```python
from build123d import *

# Parameters (mm, degrees)
SKETCH1_W           = 25
SKETCH1_H           = 35
SKETCH1_R           = 4
BOSS_EXTRUDE1_DEPTH = 6
FILLET1_R           = 12.5
SKETCH2_R           = 20
CUT_EXTRUDE1_DEPTH  = 6


with BuildPart() as part:
    # Sketch1 → Boss-Extrude1 (new body)
    with BuildSketch(Plane(origin=(0, 0, 0), x_dir=(1, 0, 0), z_dir=(0, 1, 0))):
        with Locations((12.5, 17.5)):
            Rectangle(SKETCH1_W, SKETCH1_H)
        with Locations(Location((12.5, 25, 0), (0, 0, 270))):
            Circle(SKETCH1_R, mode=Mode.SUBTRACT)
    extrude(amount=BOSS_EXTRUDE1_DEPTH)

    # Fillet1
    fillet1_edges = [part.edges().sort_by_distance(p)[0] for p in [
        (25, 3, -35),
        (0, 3, -35),
    ]]
    fillet(fillet1_edges, radius=FILLET1_R - 0.0001)  # a hair under: the kernel refuses the full size

    # Sketch2 → Cut-Extrude1 (cut)
    with BuildSketch(Plane(origin=(0, 6, 0), x_dir=(1, 0, 0), z_dir=(0, 1, 0))):
        with Locations((12.5, -12)):
            Circle(SKETCH2_R)
    extrude(amount=-CUT_EXTRUDE1_DEPTH, mode=Mode.SUBTRACT)


solid = part.part
```
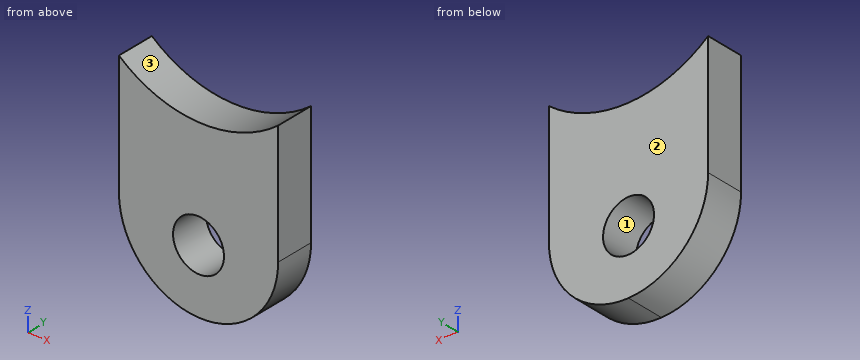
Read the model definition and answer for the solid it produces. Units are mm, in the model's axes. Face numbers are marked on the shaded views. Round coordinates to 2 decimals unless told otherwise and drop trailing zeros. Loops run counter-clockwise (first coordinate to the right, second up) from the corner with the lowest first, then second, coordinate; pieces in that order, holes last. Notation, with made-up numbers: (84, 7.5) -> (132, 7.5) arc R27 ccw to (132, 27.5) -> close; hole circle Ø9 at (6.5, 59). An arc over 180 degrees is marked (long way). One line per item, written item: value.
1) The mould has two halves that part along Z. Classify the marked faces 1, 2 and 3: pulls with the +Z half, pulls with the -Z half, needs draft (parallel to the pull), parting line crosses it, or undercut.
Answer list:
face 1: undercut
face 2: needs draft
face 3: pulls with the +Z half
2) A cutting plane is placed at D-D (x = 18.25). Determine the outline of the cut face in (y, z).
Answer list:
outline: (0, -33.6) -> (6, -33.6) -> (6, -7.16) -> (0, -7.16) -> close
3) A cutting plane is placed at B-B (z = -24). Determine the outline of the cut face in (x, y), and give its area (3 significant figures).
Answer list:
outline: (0.09, 0) -> (8.63, 0) -> (8.63, 6) -> (0.09, 6) -> close; (16.37, 0) -> (24.91, 0) -> (24.91, 6) -> (16.37, 6) -> close
area: 102 mm²
4) A cutting plane is placed at C-C (x = 11). Determine the outline of the cut face in (y, z), and give its area (3 significant figures).
Answer list:
outline: (0, -34.91) -> (6, -34.91) -> (6, -28.71) -> (0, -28.71) -> close; (0, -21.29) -> (6, -21.29) -> (6, -7.94) -> (0, -7.94) -> close
area: 117 mm²
5) Consider L1, parallel to Z at x = 14.25, y = 4.6; L2, parallel to X at y = 3.3, z = -25; L3, parallel to Z at x = 15.75, y = 5.65. Determine where each line is inside the solid, lowest interval first. Write a range as [from, to].
Answer list:
L1: z = [-34.88, -28.6], [-21.4, -7.92]
L2: x = [0.25, 8.5], [16.5, 24.75]
L3: z = [-34.57, -27.33], [-22.67, -7.73]
6) Flat-ended cylindrical pins translate along their axes: P1, Ø5, axis at x = 12, z = -30.5, coming from the -Y side; P2, Ø1, axis at x = 5, y = 4, coming from the -Z side; P3, Ø3, axis at x = 20.5, y = 4, coming from the +Z side; P4, Ø6.5, axis at x = 12.5, z = -25, coming from the +Y side. Find the tip coordinate at first contact, or state that the pin passes through.
Answer list:
P1: stops at y = 0
P2: stops at z = -32.86
P3: stops at z = -5.6
P4: passes through
